The model under review builds one solid part; all positions refer to its coordinate system, in mm. A direction names the side the tool comes from. Coordinates: 2 decimals unless noted, no trailing zeros. Write each loop counter-clockwise with the first axis right and the second up, starting at its lowest first coordinate (ties: lowest second). Pieces come first, ordered by that corner, then holes. Notation, with made-up numbers: (3, -8) - (26, -8) arc R13 cw to (26, 9) - close; hole circle Ø4 at (69, 6.25). An arc over 180 degrees is marked (long way). Put each result on its own line as item: value. Start each with the question number.
Item 1: For pin 1 (1.5 mm diameter, centred on y = -2, z = 4, fed in from -X); pin 2 (1.5 mm diameter, centred on y = -9, z = 5.5, fed in from -X); pin 3 (1.2 mm diameter, centred on y = -23, z = 2.5, fed in from +X), all flat-tipped, find the tip position at first contact; note any pin that passes through.
Item 2: Consider section B-B on y = -55.75. Give the boundary of the cut face in (x, z).
Item 3: Consider section A-A on z = 3.65. State how many separate pieces and enclosed holes the cut face has, then the cut area to 3 significant figures.
Item 4: Consider section D-D on x = -60.5. Give the boundary of the cut face in (y, z).
Item 5: Mouldability with a two-part tool opening along Y and no side actions: class faces 1 (the face through (-45, -20, 6)), 2 (the face through (-29, -23, 3)), 3 (the face through (-31, -21.5, 3)), 4 (the face through (-21.85, -11.99, 3.04)) as pulls with the +Y half, pulls with the -Y half, needs draft (parallel to the pull), parting line crosses it, or undercut.
Item 6: To check wall thickness, follow L1, parallel to Y at x = -91, z = 1.6; L2, parallel to Y at x = 12, z = 4.8; L3, parallel to Y at x = -13, z = 3.9. State the ranges of each line that lie inside material, in increasing order. Write a range as [from, to].
Item 7: Consider section C-C on x = -113.25. Give the boundary of the cut face in (y, z).
Item 8: Machinability: for faces 5 (the face through (-70, -15, 3)), 6 (the face through (-0.16, 14.24, 2.96)), 7 (the face through (-46, -35, 3)), which of the approach directions +Z, -Z, +X, -X, +Y, -Y give a long, thin tool a straight path to every point of the face, cutting with its end or side? Answer none if there is none.
```python
from build123d import *

# Parameters (mm, degrees)
SKETCH_1_W      = 4
SKETCH_1_H      = 2.5
SKETCH_1_R      = 1.25
SKETCH_1_R_2    = 4.75
SKETCH_1_R_3    = 1.5
EXTRUDE_1_DEPTH = 6
FILLET_1_R      = 10
FILLET_2_R      = 20
FILLET_3_R      = 10


with BuildPart() as part:
    # Эскиз1 → Бобышка-Вытянуть1 (new body)
    with BuildSketch(Plane.XY):
        with BuildLine():
            Line((19, -35), (19, 0))
            ThreePointArc((19, 0), (0, 19), (-19, 0))
            Line((-19, 0), (-19, -15))
            Line((-19, -15), (-29, -15))
            Line((-29, -15), (-29, -17.5))
            Line((-29, -17.5), (-33, -17.5))
            Line((-33, -17.5), (-33, -15))
            Line((-33, -15), (-119, -15))
            Line((-119, -15), (-119, -60))
            Line((-119, -60), (-107.5, -60))
            Line((-107.5, -60), (-97.5, -35))
            Line((-97.5, -35), (19, -35))
        make_face()
        with Locations((-31, -22.75)):
            Rectangle(SKETCH_1_W, SKETCH_1_H, mode=Mode.SUBTRACT)
        with Locations((0, -13)):
            Circle(SKETCH_1_R, mode=Mode.SUBTRACT)
        with Locations((-13, 0)):
            Circle(SKETCH_1_R, mode=Mode.SUBTRACT)
        Circle(SKETCH_1_R_2, mode=Mode.SUBTRACT)
        with Locations((13, 0)):
            Circle(SKETCH_1_R, mode=Mode.SUBTRACT)
        with Locations((0, 13)):
            Circle(SKETCH_1_R, mode=Mode.SUBTRACT)
        with Locations((-113.25, -55.75)):
            Circle(SKETCH_1_R_3, mode=Mode.SUBTRACT)
        with Locations((-113.25, -48.25)):
            Circle(SKETCH_1_R_3, mode=Mode.SUBTRACT)
    extrude(amount=EXTRUDE_1_DEPTH)

    # Скругление1
    fillet_1_edges = [part.edges().sort_by_distance(p)[0] for p in [
        (-19, -15, 3),
    ]]
    fillet(fillet_1_edges, radius=FILLET_1_R - 0.0001)  # a hair under: the kernel refuses the full size

    # Скругление2
    fillet_2_edges = [part.edges().sort_by_distance(p)[0] for p in [
        (19, -35, 3),
    ]]
    fillet(fillet_2_edges, radius=FILLET_2_R)

    # Скругление3
    fillet_3_edges = [part.edges().sort_by_distance(p)[0] for p in [
        (-119, -15, 3),
        (-97.5, -35, 3),
    ]]
    fillet(fillet_3_edges, radius=FILLET_3_R)


solid = part.part
```
Report:
1. pin 1: x = -19
1. pin 2: x = -20.2
1. pin 3: x = 17.58
2. outline: (-119, 0) - (-114.75, 0) - (-114.75, 6) - (-119, 6) - close; (-111.75, 0) - (-105.8, 0) - (-105.8, 6) - (-111.75, 6) - close
3. separate pieces: 1
3. enclosed holes: 8
3. area: 4,110 mm²
4. outline: (-35, 0) - (-15, 0) - (-15, 6) - (-35, 6) - close
5. face 1: needs draft
5. face 2: undercut
5. face 3: undercut
5. face 4: pulls with the +Y half
6. L1: [-35, -15]
6. L2: [-30.2, -0.75], [0.75, 14.73]
6. L3: [-35, -1.25], [1.25, 13.86]
7. outline: (-60, 0) - (-57.25, 0) - (-57.25, 6) - (-60, 6) - close; (-54.25, 0) - (-49.75, 0) - (-49.75, 6) - (-54.25, 6) - close; (-46.75, 0) - (-15.95, 0) - (-15.95, 6) - (-46.75, 6) - close
8. face 5: +Z, -Z, -X, +Y
8. face 6: +Z, -Z
8. face 7: +Z, -Z, +X, -Y
